```python
from build123d import *

# Parameters (mm, degrees)
F0_R     = 38.1
F1_DEPTH = 12.7
F3_DEPTH = 25.4


with BuildPart() as f1:
    # F0 (on Front) → F1 (new body, symmetric)
    with BuildSketch(Plane.XZ):
        Circle(F0_R)
    extrude(amount=F1_DEPTH, both=True)

    # F2 (on face) → F3 (join)
    with BuildSketch(Plane.XZ.offset(12.7)):
        Polygon((10.9985226281, 19.05), (-10.9985226281, 19.05), (-21.9970452561, 0), (-10.9985226281, -19.05), (10.9985226281, -19.05), (21.9970452561, 0), align=None)
    extrude(amount=F3_DEPTH)


solid = f1.part
```
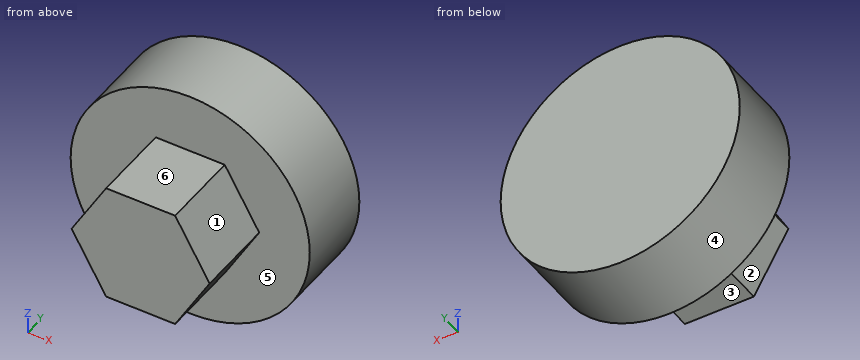
Design review of the part built by this model. Coordinates are the model's own, in mm. Face numbers are marked on the shaded views. A direction names the side the tool comes from. Give positions to 0.01 mm unless a question says otherwise; leave off trailing zeros. Order: outer loops, then holes, each group sorted by start corner. A loop starts at its lowest first (then second) coordinate and runs counter-clockwise, first axis right, second up. Notation, with made-up numbers: M 50.5,25.25 L 66.5,25.25 A27 ccw 66.5,50.25 Z; hole C 19,22.25 d10. An arc over 180 degrees is marked long. One line per question, with ' | ' between items. Start each with the question number.
Q1. We need section A-A (y = -20). Write out the cut boundary in (x, z).
Q2. The part is to be moulded in two halves that separate along X. For the marked faces 1, 2 and 3, say which applies: +X half, -X half, draft (parallel to the pull), parting line (faces both ways), or undercut.
Q3. Machinability: for the marked faces 4, 5 and 6, which of the approach directions +Z, -Z, +X, -X, +Y, -Y give a long, thin tool a straight path to every point of the face, cutting with its end or side? Answer none if there is none.
Q4. For pin 1 Ø11 at (x, y) = (-2.5, -30.5) entering from +Z; pin 2 Ø4 at (x, y) = (-21.5, -7.5) entering from -Z; pin 3 Ø1.5 at (y, z) = (-1.5, 12) entering from -X; pin 4 Ø8 at (x, z) = (5.5, -21) entering from -Y, all flat-tipped, find the tip position at first contact; note any pin that passes through.
Q5. For L1, parallel to Y at x = 27, z = -1.5; L2, parallel to Z at x = 22, y = 5; L3, parallel to Z at x = 9, y = -2, list the stretches that pass through material, from the lowest coordinate up. Write a range as [from, to].
Q6. We need section C-C (z = -9). Write out the cut boundary in (x, y).
Q7. We need section B-B (x = 0). Write out the cut boundary in (y, z), plus the area to 3 significant figures.
Q8. We need section D-D (y = -8.5). Write out the cut boundary in (x, z), plus the area to 3 significant figures.
Returned:
1) outline: M -22,0 L -11,-19.05 L 11,-19.05 L 22,0 L 11,19.05 L -11,19.05 Z
2) face 1: +X half | face 2: -X half | face 3: draft
3) face 4: +Y, -Y | face 5: -Y | face 6: +Z, +X, -X, -Y
4) pin 1: z = 19.05 | pin 2: z = -32.73 | pin 3: x = -36.4 | pin 4: y = -38.1
5) L1: [-12.7, 12.7] | L2: [-31.11, 31.11] | L3: [-37.02, 37.02]
6) outline: M -37.02,-12.7 L -16.8,-12.7 L -16.8,-38.1 L 16.8,-38.1 L 16.8,-12.7 L 37.02,-12.7 L 37.02,12.7 L -37.02,12.7 Z
7) outline: M -38.1,-19.05 L -12.7,-19.05 L -12.7,-38.1 L 12.7,-38.1 L 12.7,38.1 L -12.7,38.1 L -12.7,19.05 L -38.1,19.05 Z | area: 2,900 mm2
8) outline: C 0,0 d76.2 | area: 4,560 mm2
